```python
from build123d import *

# Parameters (mm, degrees)
F1_DEPTH = 25.4
F2_R     = 5.08
F3_R     = 5.08
F5_DEPTH = 10.16


with BuildPart() as f1:
    # F0 (on Front) → F1 (new body)
    with BuildSketch(Plane.XZ):
        Polygon((0, 38.0835495889), (0, 25.4), (-25.4, 25.4), (-27.8758880853, 25.4), (-27.8758880853, 7.62), (30.48, 7.62), (30.48, 38.1), (0, 38.1), align=None)
    extrude(amount=F1_DEPTH)

    # F2
    f2_edges = [f1.edges().sort_by_distance(p)[0] for p in [
        (0, -12.7, 25.4),
        (0, -12.7, 38.1),
        (30.48, -12.7, 38.1),
        (30.48, -12.7, 7.62),
    ]]
    fillet(f2_edges, radius=F2_R)

    # F3
    f3_edges = [f1.edges().sort_by_distance(p)[0] for p in [
        (30.48, 0, 22.86),
        (-16.477944, -25.4, 25.4),
    ]]
    fillet(f3_edges, radius=F3_R)

    # F4 (on face) → F5 (join)
    with BuildSketch(Plane(origin=(-27.8758880853, 0, 0), x_dir=(0, -1, 0), z_dir=(-1, 0, 0))):
        with BuildLine():
            Line((12.7, 11.557), (12.7, 21.463))
            ThreePointArc((12.7, 21.463), (7.747, 16.51), (12.7, 11.557))
        make_face()
        with BuildLine():
            ThreePointArc((17.653, 16.51), (16.2022998872, 20.0122998872), (12.7, 21.463))
            Line((12.7, 21.463), (12.7, 11.557))
            ThreePointArc((12.7, 11.557), (16.2022998872, 13.0077001128), (17.653, 16.51))
        make_face()
    extrude(amount=F5_DEPTH)


solid = f1.part
```
Part model, mm, in its own coordinate system. A direction names the side the tool comes from. Round coordinates to 2 decimals unless told otherwise and drop trailing zeros. Loops run counter-clockwise (first coordinate to the right, second up) from the corner with the lowest first, then second, coordinate; pieces in that order, holes last. Notation, with made-up numbers: (82.5, -34) -> (89.5, -34) arc R32 cw to (89.5, 0) -> close; hole circle Ø7 at (38, -19). An arc over 180 degrees is marked (long way). Use a Markdown table: item, result.
1) Probe line 1 (Z direction, x = -12, y = -5); line 2 (X direction, y = -19.75, z = 13.5); line 3 (Y direction, x = 5.5, z = 35). List the from-to ranges inside material, lowest first. Write a range as [from, to].
The answers:
| item | result |
|---|---|
| line 1 | z = [7.62, 25.4] |
| line 2 | x = [-27.88, 30.48] |
| line 3 | y = [-25, -0.4] |
2) Cut at C-C, the plane z = 15.5. List the corners of the cut face in (x, y).
The answers:
| item | result |
|---|---|
| outline | (-38.04, -17.55) -> (-27.88, -17.55) -> (-27.88, -25.4) -> (25.4, -25.4) arc R5.08 ccw to (30.48, -20.32) -> (30.48, -5.08) arc R5.08 ccw to (25.4, 0) -> (-27.88, 0) -> (-27.88, -7.85) -> (-38.04, -7.85) -> close |
3) Cut at B-B, the plane y = -18.5. List the corners of the cut face in (x, z).
The answers:
| item | result |
|---|---|
| outline | (-27.88, 7.62) -> (25.4, 7.62) arc R5.08 ccw to (30.48, 12.7) -> (30.48, 33.02) arc R5.08 ccw to (25.4, 38.1) -> (5.08, 38.1) arc R5.08 ccw to (0, 33.02) -> (0, 30.48) arc R5.08 cw to (-5.08, 25.4) -> (-27.88, 25.4) -> close |
4) Cut at A-A, the plane x = 24. List the corners of the cut face in (y, z).
The answers:
| item | result |
|---|---|
| outline | (-25.4, 12.7) arc R5.08 ccw to (-20.32, 7.62) -> (-5.08, 7.62) arc R5.08 ccw to (0, 12.7) -> (0, 33.02) arc R5.08 ccw to (-5.08, 38.1) -> (-20.32, 38.1) arc R5.08 ccw to (-25.4, 33.02) -> close |
5) Cut at D-D, the plane y = -11.75. List the corners of the cut face in (x, z).
The answers:
| item | result |
|---|---|
| outline | (-38.04, 11.65) -> (-27.88, 11.65) -> (-27.88, 7.62) -> (25.4, 7.62) arc R5.08 ccw to (30.48, 12.7) -> (30.48, 33.02) arc R5.08 ccw to (25.4, 38.1) -> (5.08, 38.1) arc R5.08 ccw to (0, 33.02) -> (0, 30.48) arc R5.08 cw to (-5.08, 25.4) -> (-27.88, 25.4) -> (-27.88, 21.37) -> (-38.04, 21.37) -> close |
6) Drop flat-ended pins along their axis: pin 1 Ø4 at (x, y) = (-20.5, -15) entering from +Z; pin 2 Ø4 at (x, y) = (2, -14) entering from +Z; pin 3 Ø5 at (y, z) = (-19, 24) entering from -X. Give the stop position or say it passes through.
The answers:
| item | result |
|---|---|
| pin 1 | stops at z = 25.4 |
| pin 2 | stops at z = 37.98 |
| pin 3 | stops at x = -27.88 |
7) Tool access for faces 1 (the cylindrical face through (-16.638, -23.872, 23.951)), 2 (the cylindrical face through (28.952, -1.449, 23.002)), 3 (the cylindrical face through (-16.638, -1.449, 23.872)), 4 (the flat face through (0, -13, 32)): list every direction of +Z, -Z, +X, -X, +Y, -Y with a clear straight run to the whole face (end or side of a thin tool).
The answers:
| item | result |
|---|---|
| face 1 | +Z, -X, -Y |
| face 2 | +Z, -Z, +X, +Y |
| face 3 | +Z, -X, +Y |
| face 4 | +Z, -X, +Y, -Y |
